```python
from build123d import *

# Parameters (mm, degrees)
SKETCH1_R           = 1.5
BOSS_EXTRUDE1_DEPTH = 3
LPATTERN1_COUNT     = 2
LPATTERN1_PITCH     = 15
SKETCH2_R           = 3
SKETCH2_R_2         = 1.5
BOSS_EXTRUDE2_DEPTH = 4
LPATTERN2_COUNT     = 2
LPATTERN2_PITCH     = 8
SKETCH3_W           = 30
SKETCH3_H           = 3
BOSS_EXTRUDE3_DEPTH = 15


with BuildPart() as part:
    # Sketch1 → Boss-Extrude1 (new body)
    with BuildSketch(Plane.XY):
        with BuildLine():
            Line((0, 3), (45, 3))
            ThreePointArc((45, 3), (47.298133329, 1.928362829), (47.954423259, -0.520944533))
            Line((47.954423259, -0.520944533), (44.427883645, -20.520944533))
            ThreePointArc((44.427883645, -20.520944533), (43.456627447, -22.25101053), (41.617963293, -22.996517797))
            Line((41.617963293, -22.996517797), (0.144502907, -24.996517797))
            ThreePointArc((0.144502907, -24.996517797), (-2.069600357, -24.171809006), (-3, -22))
            Line((-3, -22), (-3, 0))
            ThreePointArc((-3, 0), (-2.121320344, 2.121320344), (0, 3))
        make_face()
        with Locations((45, 0)):
            Circle(SKETCH1_R, mode=Mode.SUBTRACT)
        with Locations((41.473460386, -20)):
            Circle(SKETCH1_R, mode=Mode.SUBTRACT)
        with Locations((0, -22)):
            Circle(SKETCH1_R, mode=Mode.SUBTRACT)
        Circle(SKETCH1_R, mode=Mode.SUBTRACT)
        Polygon((3.881124623, -14.414030159), (3.881124623, -5.613630965), (6.529032345, -2.186926854), (37.60300826, -2.186926854), align=None, mode=Mode.SUBTRACT)
        Polygon((3.881124623, -19.476206686), (41.473460386, -5.845729285), (41.473460386, -15.893743297), (35.578137649, -19.476206686), align=None, mode=Mode.SUBTRACT)
    extrude(amount=BOSS_EXTRUDE1_DEPTH)


with BuildPart() as lpattern1_1:
    # LPattern1: pattern copy
    add(part.part.moved(Location(Vector(0, 0, 1) * (1 * LPATTERN1_PITCH))))


with BuildPart() as part_1:
    add(part.part)

    # Sketch2 → Boss-Extrude2 (add)
    with BuildSketch(Plane.XY.offset(3)):
        with Locations((45, 0)):
            Circle(SKETCH2_R)
        with Locations((45, 0)):
            Circle(SKETCH2_R_2, mode=Mode.SUBTRACT)
    boss_extrude2 = extrude(amount=BOSS_EXTRUDE2_DEPTH)



with BuildPart() as lpattern1_1_1:
    add(lpattern1_1.part)

    # LPattern2: Boss-Extrude2 ×2
    with Locations(*[(0, 0, i * LPATTERN2_PITCH) for i in range(1, LPATTERN2_COUNT)]):
        add(boss_extrude2)


with BuildPart() as part_2:
    add(part_1.part)

    add(lpattern1_1_1.part)  # Boss-Extrude3 merges LPattern1_1
    # Sketch3 → Boss-Extrude3 (add)
    with BuildSketch(Plane.XY.offset(3)):
        with Locations((25, 1.5)):
            Rectangle(SKETCH3_W, SKETCH3_H)
    extrude(amount=BOSS_EXTRUDE3_DEPTH)


solid = part_2.part
```
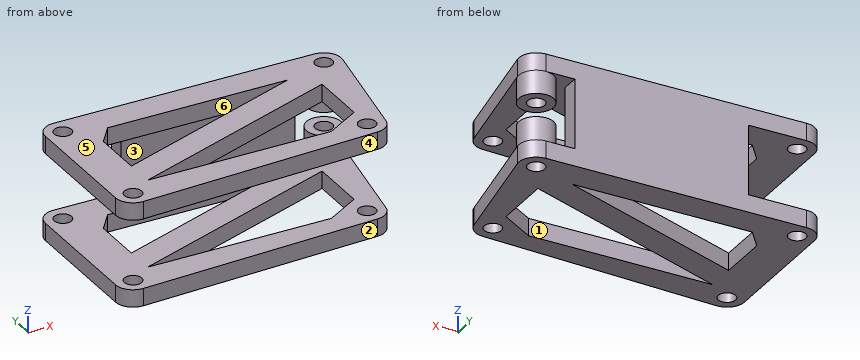
CAD build for the part. Positions are in the model's coordinates, mm. Face numbers are marked on the shaded views. A direction names the side the tool comes from. Give positions to 0.01 mm unless a question says otherwise; leave off trailing zeros. Order: outer loops, then holes, each group sorted by start corner. A loop starts at its lowest first (then second) coordinate and runs counter-clockwise, first axis right, second up.
(1) Drill centre lines: L1, parallel to Y at x = 0, z = 16.75; L2, parallel to Z at x = 3, y = -5.5; L3, parallel to Y at x = 45, z = 4. Where is each one in solid material? Low to high.
(2) Mould opens along X. For the marked faces 4, 5 and 6 say: released by +X, released by -X, zero draft, split by the parting line, or undercut.
(3) Saw through at A-A, the plane z = 3.5. Give the cut face in (x, y).
(4) Saw through at C-C, the plane x = 23.5. Give the cut face in (y, z).
(5) Flat gauge pins, fed straight in: pin 1 (3.5 mm diameter, centred on x = 25, z = 9.5, fed in from -Y); pin 2 (1.5 mm diameter, centred on y = 2, z = 11.5, fed in from -X); pin 3 (0.9 mm diameter, centred on x = 24, z = 1, fed in from -Y); pin 4 (2 mm diameter, centred on x = 34.5, y = -16.5, fed in from -Z) (3 decimals). Where does each tip first touch, or does it go through?
(6) Tool access for the marked faces 1, 2 and 3: list every direction of +Z, -Z, +X, -X, +Y, -Y with a clear straight run to the whole face (end or side of a thin tool).
(7) Saw through at B-B, the plane y = -10.5. Give the cut face in (x, z).
(8) Saw through at D-D, the plane y = -20. Give the cut face in (x, z).
Results found:
1. L1: y = -25 to -23.5, -20.5 to -1.5, 1.5 to 3
1. L2: z = 0 to 3, 15 to 18
1. L3: y = -3 to -1.5, 1.5 to 3
2. face 4: released by +X
2. face 5: zero draft
2. face 6: undercut
3. outline: (10, 0) - (40, 0) - (40, 3) - (10, 3) - close; circle Ø6 at (45, 0); hole circle Ø3 at (45, 0)
4. outline: (-23.87, 0) - (-19.48, 0) - (-19.48, 3) - (-23.87, 3) - close; (-23.87, 15) - (-19.48, 15) - (-19.48, 18) - (-23.87, 18) - close; (-12.36, 0) - (-7.3, 0) - (-7.3, 3) - (-12.36, 3) - close; (-12.36, 15) - (-7.3, 15) - (-7.3, 18) - (-12.36, 18) - close; (-2.19, 0) - (3, 0) - (3, 18) - (-2.19, 18) - (-2.19, 15) - (0, 15) - (0, 3) - (-2.19, 3) - close
5. pin 1: stops at y = 0
5. pin 2: stops at x = 10
5. pin 3: stops at y = -23.87
5. pin 4: passes through
6. face 1: +Z, -Z
6. face 2: +Z, -Z, +X, -Y
6. face 3: -X, -Y
7. outline: (-3, 0) - (3.88, 0) - (3.88, 3) - (-3, 3) - close; (-3, 15) - (3.88, 15) - (3.88, 18) - (-3, 18) - close; (14.68, 0) - (28.64, 0) - (28.64, 3) - (14.68, 3) - close; (14.68, 15) - (28.64, 15) - (28.64, 18) - (14.68, 18) - close; (41.47, 0) - (46.19, 0) - (46.19, 3) - (41.47, 3) - close; (41.47, 15) - (46.19, 15) - (46.19, 18) - (41.47, 18) - close
8. outline: (-3, 0) - (39.97, 0) - (39.97, 3) - (-3, 3) - close; (-3, 15) - (39.97, 15) - (39.97, 18) - (-3, 18) - close; (42.97, 0) - (44.52, 0) - (44.52, 3) - (42.97, 3) - close; (42.97, 15) - (44.52, 15) - (44.52, 18) - (42.97, 18) - close
